Autodesk Inventor part; units mm, degrees
ref_plane "YZ Plane" through (0, 0, 0) normal (1, 0, 0) x (0, 1, 0)
ref_plane "XZ Plane" through (0, 0, 0) normal (0, 1, 0) x (-1, 0, 0)
ref_plane "XY Plane" through (0, 0, 0) normal (0, 0, 1) x (1, 0, 0)
sketch "Skizze1" plane through (0, 0, 0) normal (0, 0, 1) x (1, 0, 0)
  line L0 (147.1952, 0) -> (147.1952, 200)
  line L1 (147.1952, 200) -> (0, 200)
  line L2 (0, 200) -> (0, 0)
  line L3 (0, 0) -> (-24.1421, 0)
  line L4 (-24.1421, 0) -> (-126.4024, 0)
  line L5 (-126.4024, 0) -> (-126.4024, -100)
  line L6 (-126.4024, -100) -> (273.5976, -100)
  line L7 (273.5976, -100) -> (273.5976, 0)
  line L8 (273.5976, 0) -> (171.3373, 0)
  line L9 (171.3373, 0) -> (147.1952, 0)
  circle A0 centre (223.5976, -50) radius 10
  circle A1 centre (-76.4024, -50) radius 10
  circle A2 centre (73.5976, -50) radius 10
  dimension "d34" = 20
  dimension "d35" = 90
  dimension "d36" = 90
  dimension "d37" = 90
  dimension "d38" = 126.4024
  dimension "d39" = 273.5976
  dimension "d40" = 400
  dimension "d41" = 200
  dimension "d42" = 100
  dimension "d43" = 0
  dimension "d44" = 0
  dimension "d45" = 0
  dimension "d46" = 0
  dimension "d47" = 0
  dimension "d48" = 100
  dimension "d49" = 0
  dimension "d50" = 50
  dimension "d51" = 50
  dimension "d52" = 102.2603
  dimension "d53" = 102.2603
  dimension "d54" = 200
  dimension "d55" = 126.4024
  dimension "d56" = 0
  dimension "d57" = 126.4024
  dimension "d58" = 200
  dimension "d59" = 50
  dimension "d60" = 200
  dimension "d61" = 273.5976
  dimension "d62" = 0
  dimension "d63" = 273.5976
  dimension "d64" = 297.7397
  dimension "d65" = 297.7397
  dimension "d66" = 350
  dimension "d67" = 50
  dimension "d68" = 0
  dimension "d69" = 400
  dimension "d70" = 100
  dimension "d71" = 400
extrude "Extrusion1" add sketch "Skizze1" along normal blind 10
sketch "Skizze2" plane through (0, 0, 10) normal (0, 0, 1) x (1, 0, 0)
  arc A0 (63.5977, 176.2843) -> (83.5977, 176.2843) centre (73.5977, 148) ccw
  line L0 (147.1952, 200) -> (0, 200)
  line L1 (147.1952, 0) -> (147.1952, 200)
  line L2 (63.5977, 183) -> (83.5977, 183)
  line L3 (83.5977, 183) -> (83.5977, 176.2843)
  line L4 (63.5977, 176.2843) -> (63.5977, 183)
  circle A1 centre (39.5977, 148) radius 2.75
  circle A2 centre (107.5977, 148) radius 2.75
  point P0 (0, 0)
  dimension "d72" = 60
  dimension "d73" = 52
  dimension "d74" = 73.5975
  dimension "d75" = 35
  dimension "d76" = 20
  dimension "d77" = 83.5975
  dimension "d78" = 5.5
  dimension "d79" = 5.5
  dimension "d80" = 52
  dimension "d81" = 68
  dimension "d82" = 0
  dimension "d83" = 39.5975
extrude "Extrusion2" cut sketch "Skizze2" against normal through all
properties part number "InnenUnten"
Source: CAD feature listing. Evaluate the final solid. Frame: model axes, mm. A direction names the side the tool comes from. Round coordinates to 2 decimals unless told otherwise and drop trailing zeros. Loops run counter-clockwise (first coordinate to the right, second up) from the corner with the lowest first, then second, coordinate; pieces in that order, holes last. Notation, with made-up numbers: (43.25, 6) - (82.25, 6) arc R10 ccw to (82.25, 20) - close; hole circle Ø11 at (46.25, 69.25). An arc over 180 degrees is marked (long way). Write item = value, one per line. Start each with the question number.
(1) Pull-direction query (Y, two-part tool) for faces 5 (the face through (75, 200, 5)), 6 (the face through (71, 19, 0)), 7 (the face through (72.421, 118.023, 5.07)); classes: +Y half, -Y half, draft (parallel to the pull), parting line (faces both ways), or undercut.
(2) Section query D-D, the plane x = -37. Output: boundary loops of the cut face in (y, z), plus the area to 3 significant figures.
(3) Section query A-A, the plane z = 1.75. Output: boundary loops of the cut face in (x, y), plus the area to 3 significant figures.
(4) Ray query, line 1 along X through (y, z) = (148, 5); line 2 along X through (y, z) = (177, 3); line 3 along Y through (x, z) = (-63, 6.5). Return the intervals inside material, ascending. Write a range as from..to.
(5) Section query C-C, the plane y = -50. Output: boundary loops of the cut face in (x, z), plus the area to 3 significant figures.
(6) Set-up query: faces 1 (the face through (-62, 0, 5)), 2 (the face through (73, 183, 5)), 3 (the face through (71, 19, 10)), 4 (the face through (147.195, 99, 5)). Return all of +Z, -Z, +X, -X, +Y, -Y with unobstructed straight access to the full face (end or side cutting, diameter ignored); none if empty.
(7) Section query B-B, the plane x = -80. Output: boundary loops of the cut face in (y, z).
(8) Pin query (flat end, axial travel): pin 1 (3 mm diameter, centred on y = 85.5, z = 6, fed in from -X); pin 2 (5 mm diameter, centred on x = 197.5, z = 6, fed in from +Y); pin 3 (16 mm diameter, centred on x = 223.6, y = -50, fed in from -Z); pin 4 (3.5 mm diameter, centred on y = 180, z = 3, fed in from +X). Return the tip coordinate at first contact, or that it passes through.
Conclusion:
q1.face_5 = +Y half
q1.face_6 = draft
q1.face_7 = undercut
q2.outline = (-100, 0) - (0, 0) - (0, 10) - (-100, 10) - close
q2.area = 1,000 mm2
q3.outline = (-126.4, -100) - (273.6, -100) - (273.6, 0) - (147.2, 0) - (147.2, 200) - (0, 200) - (0, 0) - (-126.4, 0) - close; hole circle Ø20 at (-76.4, -50); hole circle Ø5.5 at (39.6, 148); hole circle Ø20 at (73.6, -50); hole (63.6, 176.28) arc R30 ccw (long way) to (83.6, 176.28) - (83.6, 183) - (63.6, 183) - close; hole circle Ø5.5 at (107.6, 148); hole circle Ø20 at (223.6, -50)
q3.area = 65,500 mm2
q4.line_1 = 0..36.85, 42.35..43.6, 103.6..104.85, 110.35..147.2
q4.line_2 = 0..63.6, 83.6..147.2
q4.line_3 = -100..0
q5.outline = (-126.4, 0) - (-86.4, 0) - (-86.4, 10) - (-126.4, 10) - close; (-66.4, 0) - (63.6, 0) - (63.6, 10) - (-66.4, 10) - close; (83.6, 0) - (213.6, 0) - (213.6, 10) - (83.6, 10) - close; (233.6, 0) - (273.6, 0) - (273.6, 10) - (233.6, 10) - close
q5.area = 3,400 mm2
q6.face_1 = +Z, -Z, -X, +Y
q6.face_2 = +Z, -Z
q6.face_3 = +Z, +X, -X, +Y, -Y
q6.face_4 = +Z, -Z, +X, +Y
q7.outline = (-100, 0) - (-59.33, 0) - (-59.33, 10) - (-100, 10) - close; (-40.67, 0) - (0, 0) - (0, 10) - (-40.67, 10) - close
q8.pin_1 = 0
q8.pin_2 = 0
q8.pin_3 = through
q8.pin_4 = 147.2
